```python
from build123d import *

# Parameters (mm, degrees)
RESSALTO_EXTRUS_O1_DEPTH = 1000
ESBO_O2_R                = 3.5
CORTE_EXTRUS_O1_DEPTH    = 981.312123765


# Read off the part's stored shape, not the designer's step: KR25-N.step
with BuildPart() as part:
    # Esboço1 → Ressalto-extrusão1 (new body)
    with BuildSketch(Plane.ZY.offset(20)):
        with BuildLine():
            Line((0, 10), (0, -10))
            Line((0, -10), (1.5, -11.5))
            Line((1.5, -11.5), (6.0986495, -11.5))
            Line((6.0986495, -11.5), (9.898648987, -7.7))
            Line((9.898648987, -7.7), (13.280138132, -7.7))
            Line((13.280138132, -7.7), (14.509842724, -8.929704991))
            ThreePointArc((14.509842724, -8.929704991), (16.046259432, -9.658087148), (16.774641091, -11.194504091))
            Line((16.774641091, -11.194504091), (16.980137, -11.4))
            Line((16.980137, -11.4), (19.008698, -11.4))
            Line((19.008698, -11.4), (19.226365837, -11.182332163))
            ThreePointArc((19.226365837, -11.182332163), (19.953497116, -9.6580866), (21.477742889, -8.93095576))
            Line((21.477742889, -8.93095576), (21.9, -8.508698852))
            Line((21.9, -8.508698852), (21.9, 8.508698852))
            Line((21.9, 8.508698852), (21.477742889, 8.93095576))
            ThreePointArc((21.477742889, 8.93095576), (19.953497116, 9.6580866), (19.226365837, 11.182332163))
            Line((19.226365837, 11.182332163), (19.008698, 11.4))
            Line((19.008698, 11.4), (16.980137, 11.4))
            Line((16.980137, 11.4), (16.774641091, 11.194504091))
            ThreePointArc((16.774641091, 11.194504091), (16.046259432, 9.658087148), (14.509842724, 8.929704991))
            Line((14.509842724, 8.929704991), (13.280138132, 7.7))
            Line((13.280138132, 7.7), (9.898648987, 7.7))
            Line((9.898648987, 7.7), (6.0986495, 11.5))
            Line((6.0986495, 11.5), (1.5, 11.5))
            Line((1.5, 11.5), (0, 10))
        make_face()
    extrude(amount=-RESSALTO_EXTRUS_O1_DEPTH)

    # Esboço2 → Corte-extrusão1 (cut, through all)
    with BuildSketch(Plane.XY.offset(21.9)):
        with Locations((30, 0)):
            Circle(ESBO_O2_R)
        with Locations((90, 0)):
            Circle(ESBO_O2_R)
        with Locations((150, 0)):
            Circle(ESBO_O2_R)
        with Locations((210, 0)):
            Circle(ESBO_O2_R)
        with Locations((270, 0)):
            Circle(ESBO_O2_R)
        with Locations((330, 0)):
            Circle(ESBO_O2_R)
        with Locations((390, 0)):
            Circle(ESBO_O2_R)
        with Locations((450, 0)):
            Circle(ESBO_O2_R)
        with Locations((510, 0)):
            Circle(ESBO_O2_R)
        with Locations((570, 0)):
            Circle(ESBO_O2_R)
        with Locations((630, 0)):
            Circle(ESBO_O2_R)
        with Locations((690, 0)):
            Circle(ESBO_O2_R)
        with Locations((750, 0)):
            Circle(ESBO_O2_R)
        with Locations((810, 0)):
            Circle(ESBO_O2_R)
        with Locations((870, 0)):
            Circle(ESBO_O2_R)
        with Locations((930, 0)):
            Circle(ESBO_O2_R)
    extrude(amount=-CORTE_EXTRUS_O1_DEPTH, mode=Mode.SUBTRACT)


solid = part.part
```
Build history of the part. All positions in model axes, mm. Round coordinates to 2 decimals unless told otherwise and drop trailing zeros. Loops run counter-clockwise (first coordinate to the right, second up) from the corner with the lowest first, then second, coordinate; pieces in that order, holes last. Notation, with made-up numbers: M 56,15 L 87,15 A15 cw 87,22 Z; hole C 29.5,45.25 d10. An arc over 180 degrees is marked long. Answer as CSV lines item,"result".
1. Wall check: probe 1 along Y at (x, z) = (930, 9); probe 2 along Y at (x, z) = (151, 7.5); probe 3 along Y at (x, z) = (647, 12). Give the ranges that are in metal, low to high. Write a range as [from, to].
Resolved:
probe 1,"y = [-8.6, -3.5], [3.5, 8.6]"
probe 2,"y = [-10.1, -3.35], [3.35, 10.1]"
probe 3,"y = [-7.7, 7.7]"
2. Cut at A-A on x = 122.5. Write the cut outline in (y, z), then the cut area to 3 significant figures.
Resolved:
outline,"M -11.5,1.5 L -10,0 L 10,0 L 11.5,1.5 L 11.5,6.1 L 7.7,9.9 L 7.7,13.28 L 8.93,14.51 A2.53 cw 11.19,16.77 L 11.4,16.98 L 11.4,19.01 L 11.18,19.23 A2.53 cw 8.93,21.48 L 8.51,21.9 L -8.51,21.9 L -8.93,21.48 A2.53 cw -11.18,19.23 L -11.4,19.01 L -11.4,16.98 L -11.19,16.77 A2.53 cw -8.93,14.51 L -7.7,13.28 L -7.7,9.9 L -11.5,6.1 Z"
area,"433 mm²"
3. Flat gauge pins, fed straight in: P1, Ø5, axis at x = 272.5, z = 9, coming from the +Y side; P2, Ø0.6, axis at x = 514.5, z = 18, coming from the +Y side; P3, Ø5, axis at x = 688.5, z = 16, coming from the -Y side. Where does each tip first touch, or does it go through?
Resolved:
P1,"stops at y = 11.1"
P2,"stops at y = 11.4"
P3,"stops at y = -11.4"
